```python
from build123d import *

# Parameters (mm, degrees)
BOSS_EXTRUDE1_DEPTH = 3
SKETCH2_W           = 61.538461538
SKETCH2_H           = 12
BOSS_EXTRUDE2_DEPTH = 3
FILLET1_R           = 2


with BuildPart() as part:
    # Sketch1 → Boss-Extrude1 (new body)
    with BuildSketch(Plane(origin=(0, 0, 0), x_dir=(1, 0, 0), z_dir=(0, 1, 0))):
        with BuildLine():
            Line((18.124260355, -19.786982249), (29.065088757, -19.786982249))
            ThreePointArc((29.065088757, -19.786982249), (30.47930232, -19.201195811), (31.065088757, -17.786982249))
            Line((31.065088757, -17.786982249), (31.065088757, 5.213017751))
            Line((31.065088757, 5.213017751), (-30.473372781, 5.213017751))
            Line((-30.473372781, 5.213017751), (-30.473372781, -17.786982249))
            ThreePointArc((-30.473372781, -17.786982249), (-29.887586343, -19.201195811), (-28.473372781, -19.786982249))
            Line((-28.473372781, -19.786982249), (-18.715976331, -19.786982249))
            ThreePointArc((-18.715976331, -19.786982249), (-17.301762769, -20.372768686), (-16.715976331, -21.786982249))
            Line((-16.715976331, -21.786982249), (-16.715976331, -31.786982249))
            ThreePointArc((-16.715976331, -31.786982249), (-17.301762769, -33.201195811), (-18.715976331, -33.786982249))
            Line((-18.715976331, -33.786982249), (-28.473372781, -33.786982249))
            ThreePointArc((-28.473372781, -33.786982249), (-29.887586343, -34.372768686), (-30.473372781, -35.786982249))
            Line((-30.473372781, -35.786982249), (-30.473372781, -41.786982249))
            ThreePointArc((-30.473372781, -41.786982249), (-29.887586343, -43.201195811), (-28.473372781, -43.786982249))
            Line((-28.473372781, -43.786982249), (29.065088757, -43.786982249))
            ThreePointArc((29.065088757, -43.786982249), (30.47930232, -43.201195811), (31.065088757, -41.786982249))
            Line((31.065088757, -41.786982249), (31.065088757, -35.786982249))
            ThreePointArc((31.065088757, -35.786982249), (30.47930232, -34.372768686), (29.065088757, -33.786982249))
            Line((29.065088757, -33.786982249), (18.124260355, -33.786982249))
            ThreePointArc((18.124260355, -33.786982249), (16.710046793, -33.201195811), (16.124260355, -31.786982249))
            Line((16.124260355, -31.786982249), (16.124260355, -21.786982249))
            ThreePointArc((16.124260355, -21.786982249), (16.710046793, -20.372768686), (18.124260355, -19.786982249))
        make_face()
    extrude(amount=BOSS_EXTRUDE1_DEPTH)

    # Sketch2 → Boss-Extrude2 (add)
    with BuildSketch(Plane(origin=(0, 0, -5.213017751), x_dir=(-1, 0, 0), z_dir=(0, 0, -1))):
        with Locations((-0.295857988, 6)):
            Rectangle(SKETCH2_W, SKETCH2_H)
    extrude(amount=BOSS_EXTRUDE2_DEPTH)

    # Fillet1
    fillet1_edges = [part.edges().sort_by_distance(p)[0] for p in [
        (0.295857988, 0, -8.213017751),
    ]]
    fillet(fillet1_edges, radius=FILLET1_R)


solid = part.part
```
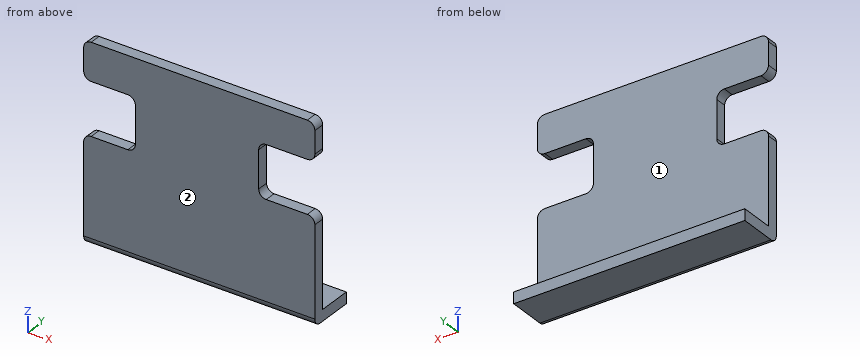
Build history of the part. All positions in model axes, mm. Face numbers are marked on the shaded views. A direction names the side the tool comes from. Give positions to 0.01 mm unless a question says otherwise; leave off trailing zeros. Loops run counter-clockwise (first coordinate to the right, second up) from the corner with the lowest first, then second, coordinate; pieces in that order, holes last.
1) Drop flat-ended pins along their axis: P1, Ø6, axis at x = -6, z = 36, coming from the +Y side; P2, Ø0.9, axis at y = 2, z = 26.5, coming from the -X side; P3, Ø1, axis at x = 6, y = 7.5, coming from the +Z side. Give the stop position or say it passes through.
Values follow:
P1: stops at y = 3
P2: stops at x = -16.72
P3: stops at z = -5.21
2) Band-saw the part on B-B on x = 3. List the corners of the cut face in (y, z).
Values follow:
outline: (0, -6.21) arc R2 ccw to (2, -8.21) - (12, -8.21) - (12, -5.21) - (3, -5.21) - (3, 43.79) - (0, 43.79) - close
3) Band-saw the part on A-A on x = -20.5. List the corners of the cut face in (y, z).
Values follow:
outline: (0, -6.21) arc R2 ccw to (2, -8.21) - (12, -8.21) - (12, -5.21) - (3, -5.21) - (3, 19.79) - (0, 19.79) - close; (0, 33.79) - (3, 33.79) - (3, 43.79) - (0, 43.79) - close
4) 3-axis set-ups, long thin cutter, end or side, ignore diameter. For the marked faces 1 and 2: which of +Z, -Z, +X, -X, +Y, -Y reach the whole face in a straight line?
Values follow:
face 1: +Z, +X, -X, +Y
face 2: +Z, -Z, +X, -X, -Y
5) Band-saw the part on C-C on y = 7.25. List the corners of the cut face in (x, z), then the cut area to 3 significant figures.
Values follow:
outline: (-30.47, -8.21) - (31.07, -8.21) - (31.07, -5.21) - (-30.47, -5.21) - close
area: 185 mm2
6) Band-saw the part on D-D on z = -1. List the corners of the cut face in (x, y), then the cut area to 3 significant figures.
Values follow:
outline: (-30.47, 0) - (31.07, 0) - (31.07, 3) - (-30.47, 3) - close
area: 185 mm2
7) Probe line 1 along Z through (x, y) = (-10, 8); line 2 along Y through (x, z) = (-7.5, 40); line 3 along Z through (x, y) = (-18, 1.25). List the from-to ranges inside material, lowest first.
Values follow:
line 1: z = -8.21 to -5.21
line 2: y = 0 to 3
line 3: z = -8.07 to 19.92, 33.65 to 43.79
